```python
from build123d import *

# Parameters (mm, degrees)
SKETCH1_R           = 2.5
BOSS_EXTRUDE1_DEPTH = 10
SKETCH2_R           = 11
SKETCH2_R_2         = 10
SKETCH2_R_3         = 6.5
SKETCH2_R_4         = 5.5
CUT_EXTRUDE1_DEPTH  = 1
FILLET1_R           = 1


with BuildPart() as part:
    # Sketch1 → Boss-Extrude1 (new body)
    with BuildSketch(Plane.XY):
        Polygon((0, 0), (50, 0), (50, 10), (40, 10), (40, 40), (10, 40), (10, 10), (0, 10), align=None)
        with Locations((25, 25)):
            Circle(SKETCH1_R, mode=Mode.SUBTRACT)
    extrude(amount=BOSS_EXTRUDE1_DEPTH)

    # Sketch2 → Cut-Extrude1 (cut)
    # profile 1 of 2: a face of its own
    with BuildSketch(Plane.XY.offset(10)):
        with Locations((25, 25)):
            Circle(SKETCH2_R)
        with Locations((25, 25)):
            Circle(SKETCH2_R_2, mode=Mode.SUBTRACT)
    # profile 2 of 2: a face of its own
    with BuildSketch(Plane.XY.offset(10)):
        with Locations((25, 25)):
            Circle(SKETCH2_R_3)
        with Locations((25, 25)):
            Circle(SKETCH2_R_4, mode=Mode.SUBTRACT)
    cut_extrude1 = extrude(amount=-CUT_EXTRUDE1_DEPTH, mode=Mode.SUBTRACT)

    # Mirror1: Cut-Extrude1 across plane
    add(cut_extrude1.mirror(Plane.XY.offset(5)), mode=Mode.SUBTRACT)

    # Fillet1
    fillet1_edges = [part.edges().sort_by_distance(p)[0] for p in [
        (45, 10, 0),
        (50, 5, 0),
        (25, 0, 0),
        (0, 5, 0),
        (50, 5, 10),
        (45, 10, 10),
        (40, 25, 10),
        (25, 40, 10),
        (10, 25, 10),
        (14, 25, 10),
        (5, 10, 10),
        (14, 25, 0),
        (0, 5, 10),
        (5, 10, 0),
        (25, 0, 10),
        (10, 25, 0),
        (25, 40, 0),
        (40, 25, 0),
    ]]
    fillet(fillet1_edges, radius=FILLET1_R - 0.0001)  # a hair under: the kernel refuses the full size


solid = part.part
```
Source: CAD feature listing. Evaluate the final solid. Frame: model axes, mm. A direction names the side the tool comes from. Round coordinates to 2 decimals unless told otherwise and drop trailing zeros. Loops run counter-clockwise (first coordinate to the right, second up) from the corner with the lowest first, then second, coordinate; pieces in that order, holes last. Notation, with made-up numbers: M -11,0.5 L 21,0.5 A11 cw 21,13.5 Z; hole C -27,0 d11. An arc over 180 degrees is marked long. Use a Markdown table: item, result. Add a question column.
1. Cut plane B-B, the plane x = 7.5. Output: boundary loops of the cut face in (y, z), and give its area (3 significant figures).
2. Pull-direction query (Y, two-part tool) for faces 1 (the cylindrical face through (44.423, 9.699, 9.715)), 2 (the flat face through (40, 25, 5)), 3 (the cylindrical face through (34.54, 28, 9.51)), 4 (the cylindrical face through (25.35, 0.285, 9.699)); classes: +Y half, -Y half, draft (parallel to the pull), parting line (faces both ways), or undercut.
3. Cut plane C-C, the plane y = 12. Output: boundary loops of the cut face in (x, z).
4. Contact query for flat-ended pins moving along their axis: pin 1 (2.5 mm diameter, centred on y = 26, z = 5.5, fed in from -X); pin 2 (2.5 mm diameter, centred on x = 2.5, z = 3, fed in from +Y); pin 3 (4 mm diameter, centred on y = 24.5, z = 3.5, fed in from +X). Output: stop coordinate, or through.
5. Set-up query: faces 5 (the cylindrical face through (44.423, 9.699, 0.285)), 6 (the cylindrical face through (5.423, 9.699, 9.715)), 7 (the cylindrical face through (30.246, 26.652, 9.507)). Return all of +Z, -Z, +X, -X, +Y, -Y with unobstructed straight access to the full face (end or side cutting, diameter ignored); none if empty.
6. Cut plane A-A, the plane z = 6.75. Output: boundary loops of the cut face in (x, y), and give its area (3 significant figures).
7. Ray query, line 1 along Y through (x, z) = (34, 9.25); line 2 along X through (y, z) = (17.5, 4); line 3 along Y through (x, z) = (7.5, 5.25). Return the intervals inside material, ascending. Write a range as [from, to].
Solution:
| question | item | result |
|---|---|---|
| 1 | outline | M 0,1 A1 ccw 1,0 L 9,0 A1 ccw 10,1 L 10,9 A1 ccw 9,10 L 1,10 A1 ccw 0,9 Z |
| 1 | area | 99.1 mm2 |
| 2 | face 1 | +Y half |
| 2 | face 2 | draft |
| 2 | face 3 | undercut |
| 2 | face 4 | -Y half |
| 3 | outline | M 10,1 A1 ccw 11,0 L 39,0 A1 ccw 40,1 L 40,9 A1 ccw 39,10 L 11,10 A1 ccw 10,9 Z |
| 4 | pin 1 | stops at x = 10 |
| 4 | pin 2 | stops at y = 10 |
| 4 | pin 3 | stops at x = 40 |
| 5 | face 5 | -Z, +X, +Y |
| 5 | face 6 | +Z, -X, +Y |
| 5 | face 7 | +Z |
| 6 | outline | M 0,0 L 50,0 L 50,10 L 40,10 L 40,40 L 10,40 L 10,10 L 0,10 Z; hole C 25,25 d5 |
| 6 | area | 1,380 mm2 |
| 7 | line 1 | y = [0.03, 18.62], [20.64, 29.36], [31.38, 39.97] |
| 7 | line 2 | x = [10, 40] |
| 7 | line 3 | y = [0, 10] |
